Work out the finished part from the listing and answer in its coordinate system (mm). A direction names the side the tool comes from. Round coordinates to 2 decimals unless told otherwise and drop trailing zeros. Write each loop counter-clockwise with the first axis right and the second up, starting at its lowest first coordinate (ties: lowest second). Pieces come first, ordered by that corner, then holes. Notation, with made-up numbers: M 85,8 L 99,8 A32 cw 99,44 Z; hole C -27,51.25 d2. An arc over 180 degrees is marked long. Answer in a Markdown table with one row per item.
```python
from build123d import *

# Parameters (mm, degrees)
SKETCH2_R           = 4
BOSS_EXTRUDE1_DEPTH = 15
SKETCH3_R           = 7.5
CUT_EXTRUDE1_DEPTH  = 2
SKETCH4_R           = 1.6
CUT_EXTRUDE2_DEPTH  = 32.591137998
CHAMFER1_SIZE       = 1
FILLET1_R           = 0.3


with BuildPart() as part:
    # Sketch2 → Boss-Extrude1 (new, symmetric)
    with BuildSketch(Plane.XY):
        Polygon((6, 1), (-6, 1), (-7, 0), (-17, 0), (-17, 6), (-16, 7), (-16, 18), (-9, 18), (-5, 22), (5, 22), (9, 18), (16, 18), (16, 7), (17, 6), (17, 0), (7, 0), align=None)
        with Locations((0, 11)):
            Circle(SKETCH2_R, mode=Mode.SUBTRACT)
    extrude(amount=BOSS_EXTRUDE1_DEPTH, both=True)

    # Sketch3 → Cut-Extrude1 (cut)
    with BuildSketch(Plane(origin=(0, 0, -15), x_dir=(-1, 0, 0), z_dir=(0, 0, -1))):
        with Locations((0, 11)):
            Circle(SKETCH3_R)
    cut_extrude1 = extrude(amount=-CUT_EXTRUDE1_DEPTH, mode=Mode.SUBTRACT)

    # Mirror1: Cut-Extrude1 across plane
    add(cut_extrude1.mirror(Plane.XY), mode=Mode.SUBTRACT)

    # Sketch4 → Cut-Extrude2 (cut, through all)
    with BuildSketch(Plane(origin=(0, 0, 0), x_dir=(-1, 0, 0), z_dir=(0, -1, 0))):
        with Locations(Location((-12, 9, 0), (0, 0, 180))):
            Circle(SKETCH4_R)
        with Locations(Location((12, 9, 0), (0, 0, 90))):
            Circle(SKETCH4_R)
        with Locations(Location((-12, -9, 0), (0, 0, 180))):
            Circle(SKETCH4_R)
        with Locations(Location((12, -9, 0), (0, 0, 90))):
            Circle(SKETCH4_R)
    extrude(amount=-CUT_EXTRUDE2_DEPTH, mode=Mode.SUBTRACT)

    # Chamfer1
    chamfer1_edges = [part.edges().sort_by_distance(p)[0] for p in [
        (-17, 0, 0),
        (17, 0, 0),
    ]]
    chamfer(chamfer1_edges, length=CHAMFER1_SIZE)

    # Fillet1
    fillet1_edges = [part.edges().sort_by_distance(p)[0] for p in [
        (-16, 18, 0),
        (-9, 18, 0),
        (-5, 22, 0),
        (5, 22, 0),
        (9, 18, 0),
        (16, 18, 0),
        (-4, 11, -13),
        (7.5, 11, -15),
        (7.5, 11, 15),
        (-4, 11, 13),
    ]]
    fillet(fillet1_edges, radius=FILLET1_R)


solid = part.part
```
1. Determine the mould class of faces 1 (the flat face through (0, 22, 0)), 2 (the cylindrical face through (1.63, 3.68, 13.86)), 3 (the cylindrical face through (-0.521, 14.966, -0.178)), 4 (the cylindrical face through (-12.97, 8.87, -7.73)) for opening direction Y: released by +Y, released by -Y, zero draft, split by the parting line, or undercut.
Calculated:
| item | result |
|---|---|
| face 1 | released by +Y |
| face 2 | undercut |
| face 3 | undercut |
| face 4 | zero draft |
2. The part is cut by section B-B (z = 9). Count the separate pieces of the cut face and the enclosed holes in it, plus the area to 3 significant figures.
Calculated:
| item | result |
|---|---|
| separate pieces | 3 |
| enclosed holes | 1 |
| area | 465 mm² |
3. The part is cut by section D-D (x = 0). Determine the outline of the cut face in (y, z).
Calculated:
| item | result |
|---|---|
| outline | M 1,-15 L 3.2,-15 A0.3 ccw 3.5,-14.7 L 3.5,-13 L 6.7,-13 A0.3 ccw 7,-12.7 L 7,12.7 A0.3 ccw 6.7,13 L 3.5,13 L 3.5,14.7 A0.3 ccw 3.2,15 L 1,15 Z; M 15,-12.7 A0.3 ccw 15.3,-13 L 18.5,-13 L 18.5,-14.7 A0.3 ccw 18.8,-15 L 22,-15 L 22,15 L 18.8,15 A0.3 ccw 18.5,14.7 L 18.5,13 L 15.3,13 A0.3 ccw 15,12.7 Z |
4. Given pin 1 (1 mm diameter, centred on x = -7, y = 12.5, fed in from +Z); pin 2 (3 mm diameter, centred on y = 12.5, z = 5.5, fed in from +X); pin 3 (3 mm diameter, centred on x = 12, z = -9, fed in from -Y); pin 4 (9.5 mm diameter, centred on x = -1.5, z = -3, fed in from -Y), each flat-ended and moving along its own axis, determine where each tip first touches the part or whether it passes through.
Calculated:
| item | result |
|---|---|
| pin 1 | stops at z = 14.96 |
| pin 2 | stops at x = 16 |
| pin 3 | passes through |
| pin 4 | stops at y = 0.75 |
5. The part is cut by section C-C (x = 12). Determine the outline of the cut face in (y, z), plus the area to 3 significant figures.
Calculated:
| item | result |
|---|---|
| outline | M 0,-15 L 18,-15 L 18,-10.6 L 0,-10.6 Z; M 0,-7.4 L 18,-7.4 L 18,7.4 L 0,7.4 Z; M 0,10.6 L 18,10.6 L 18,15 L 0,15 Z |
| area | 425 mm² |
6. A tool of negligible diameter and unlimited length cuts with its end or side. For faces 5 (the flat face through (12, 18, 0)), 6 (the flat face through (-12, 18, 0)), 7 (the flat face through (-3.2, 7.8, 13)), 8 (the flat face through (0, 1, 0)), from which of +Z, -Z, +X, -X, +Y, -Y can it reach the whole face along a straight path? Write none if from no direction.
Calculated:
| item | result |
|---|---|
| face 5 | +Z, -Z, +X, +Y |
| face 6 | +Z, -Z, -X, +Y |
| face 7 | +Z |
| face 8 | +Z, -Z, -Y |
7. The part is cut by section A-A (y = 11). Determine the outline of the cut face in (x, z).
Calculated:
| item | result |
|---|---|
| outline | M -16,-15 L -7.8,-15 A0.3 ccw -7.5,-14.7 L -7.5,-13 L -4.3,-13 A0.3 ccw -4,-12.7 L -4,12.7 A0.3 ccw -4.3,13 L -7.5,13 L -7.5,14.7 A0.3 ccw -7.8,15 L -16,15 Z; M 4,-12.7 A0.3 ccw 4.3,-13 L 7.5,-13 L 7.5,-14.7 A0.3 ccw 7.8,-15 L 16,-15 L 16,15 L 7.8,15 A0.3 ccw 7.5,14.7 L 7.5,13 L 4.3,13 A0.3 ccw 4,12.7 Z; hole C -12,-9 d3.2; hole C -12,9 d3.2; hole C 12,-9 d3.2; hole C 12,9 d3.2 |
8. Consider line 1 along Z through (x, y) = (12, 4); line 2 along Z through (x, y) = (12.5, 7.5); line 3 along Y through (x, z) = (0, 0). Determine where each line is inside the solid, lowest interval first. Write a range as from..to.
Calculated:
| item | result |
|---|---|
| line 1 | z = -15..-10.6, -7.4..7.4, 10.6..15 |
| line 2 | z = -15..-10.52, -7.48..7.48, 10.52..15 |
| line 3 | y = 1..7, 15..22 |
